The listing builds one solid part. Answer for the finished solid, in the listing's coordinates (mm). Give positions to 0.01 mm unless a question says otherwise; leave off trailing zeros. Write each loop counter-clockwise with the first axis right and the second up, starting at its lowest first coordinate (ties: lowest second). Pieces come first, ordered by that corner, then holes. Notation, with made-up numbers: (-26, -36) - (22, -36) arc R11 cw to (22, -29) - close; hole circle Ø10 at (53.25, 48). An arc over 180 degrees is marked (long way). Answer as CSV lines item,"result". Start each with the question number.
(1) For a pull along Y with two mould halves and no side action, classify faces 1 (the face through (18.348, 1.703, 0.285)), 2 (the face through (6.753, 10.143, 4.944)), 3 (the face through (1.652, 18.297, 9.715)), 4 (the face through (19.5, 10.1, 0.5)) as pulls with the +Y half, pulls with the -Y half, needs draft (parallel to the pull), parting line crosses it, or undercut.
(2) Find section A-A (y = 10). Write down the section's boundary in (x, z), then the cut area to 3 significant figures.
(3) Straight lines are drawn through the part: probe 1 along Y at (x, z) = (10, 4.5); probe 2 along Y at (x, z) = (12, 1.25); probe 3 along X at (y, z) = (7, 8). For each, find the intervals that lie inside material, in ascending order.
(4) This flat-tipped pin is pushed along its axis until it touches: pin 1 Ø6 at (x, y) = (10, 10) entering from -Z. Where does it stop, or does it pass through?
(5) Find section C-C (z = 7). Write down the section's boundary in (x, y).
from build123d import *

# Parameters (mm, degrees)
SKETCH_W        = 20
SKETCH_H        = 20
SKETCH_R        = 3.25
PAD_DEPTH       = 10
FILLET_R        = 4
CHAMFER_SIZE    = 1
CHAMFER001_SIZE = 1


with BuildPart() as part:
    # Sketch → Pad (new body)
    with BuildSketch(Plane.XY):
        with Locations((10, 10)):
            Rectangle(SKETCH_W, SKETCH_H)
        with Locations((10, 10)):
            Circle(SKETCH_R, mode=Mode.SUBTRACT)
    extrude(amount=PAD_DEPTH)

    # Fillet
    fillet_edges = [part.edges().sort_by_distance(p)[0] for p in [
        (0, 20, 5),
        (20, 20, 5),
        (0, 0, 5),
        (20, 0, 5),
    ]]
    fillet(fillet_edges, radius=FILLET_R)

    # Chamfer
    chamfer_edges = [part.edges().sort_by_distance(p)[0] for p in [
        (10, 20, 10),
        (1.171573, 18.828427, 10),
        (18.828427, 18.828427, 10),
        (0, 10, 10),
        (20, 10, 10),
        (1.171573, 1.171573, 10),
        (18.828427, 1.171573, 10),
        (10, 0, 10),
        (6.75, 10, 10),
    ]]
    chamfer(chamfer_edges, length=CHAMFER_SIZE)

    # Chamfer001
    chamfer001_edges = [part.edges().sort_by_distance(p)[0] for p in [
        (10, 20, 0),
        (1.171573, 18.828427, 0),
        (18.828427, 18.828427, 0),
        (0, 10, 0),
        (20, 10, 0),
        (1.171573, 1.171573, 0),
        (18.828427, 1.171573, 0),
        (10, 0, 0),
        (6.75, 10, 0),
    ]]
    chamfer(chamfer001_edges, length=CHAMFER001_SIZE)


solid = part.part
Result set:
1,face 1,"pulls with the -Y half"
1,face 2,"undercut"
1,face 3,"pulls with the +Y half"
1,face 4,"needs draft"
2,outline,"(0, 1) - (1, 0) - (5.75, 0) - (6.75, 1) - (6.75, 9) - (5.75, 10) - (1, 10) - (0, 9) - close; (13.25, 1) - (14.25, 0) - (19, 0) - (20, 1) - (20, 9) - (19, 10) - (14.25, 10) - (13.25, 9) - close"
2,area,"131 mm^2"
3,probe 1,"0 to 6.75, 13.25 to 20"
3,probe 2,"0 to 7.44, 12.56 to 20"
3,probe 3,"0 to 8.75, 11.25 to 20"
4,pin 1,"through"
5,outline,"(0, 4) arc R4 ccw to (4, 0) - (16, 0) arc R4 ccw to (20, 4) - (20, 16) arc R4 ccw to (16, 20) - (4, 20) arc R4 ccw to (0, 16) - close; hole circle Ø6.5 at (10, 10)"
